```python
from build123d import *

# Parameters (mm, degrees)
SKETCH1_W           = 60
SKETCH1_H           = 20
BOSS_EXTRUDE1_DEPTH = 2.5
SKETCH2_W           = 5
SKETCH2_H           = 20
CUT_EXTRUDE1_DEPTH  = 5
CUT_EXTRUDE2_DEPTH  = 6
CUT_EXTRUDE3_DEPTH  = 6


with BuildPart() as part:
    # Sketch1 → Boss-Extrude1 (new, symmetric)
    with BuildSketch(Plane.XY):
        Rectangle(SKETCH1_W, SKETCH1_H)
    extrude(amount=BOSS_EXTRUDE1_DEPTH, both=True)

    # Sketch2 → Cut-Extrude1 (cut)
    with BuildSketch(Plane.ZY.offset(30)):
        Rectangle(SKETCH2_W, SKETCH2_H)
        with BuildLine():
            Line((1.66, 6.5), (1.66, 3.5))
            ThreePointArc((1.66, 3.5), (0, 1.84), (-1.66, 3.5))
            Line((-1.66, 3.5), (-1.66, 6.5))
            ThreePointArc((-1.66, 6.5), (0, 8.16), (1.66, 6.5))
        make_face(mode=Mode.SUBTRACT)
        with BuildLine():
            Line((1.66, -3.5), (1.66, -6.5))
            ThreePointArc((1.66, -6.5), (0, -8.16), (-1.66, -6.5))
            Line((-1.66, -6.5), (-1.66, -3.5))
            ThreePointArc((-1.66, -3.5), (0, -1.84), (1.66, -3.5))
        make_face(mode=Mode.SUBTRACT)
    extrude(amount=-CUT_EXTRUDE1_DEPTH, mode=Mode.SUBTRACT)

    # Sketch3 → Cut-Extrude2 (cut)
    with BuildSketch(Plane(origin=(30, 0, 0), x_dir=(0, 0, -1), z_dir=(1, 0, 0))):
        with BuildLine():
            Line((2.16, 3.5), (2.16, 6.5))
            ThreePointArc((2.16, 6.5), (0, 8.66), (-2.16, 6.5))
            Line((-2.16, 6.5), (-2.16, 3.5))
            ThreePointArc((-2.16, 3.5), (0, 1.34), (2.16, 3.5))
        make_face()
        with BuildLine():
            Line((2.16, -6.5), (2.16, -3.5))
            ThreePointArc((2.16, -3.5), (0, -1.34), (-2.16, -3.5))
            Line((-2.16, -3.5), (-2.16, -6.5))
            ThreePointArc((-2.16, -6.5), (0, -8.66), (2.16, -6.5))
        make_face()
    extrude(amount=-CUT_EXTRUDE2_DEPTH, mode=Mode.SUBTRACT)

    # Sketch4 → Cut-Extrude3 (cut)
    with BuildSketch(Plane(origin=(0, 0, -2.5), x_dir=(-1, 0, 0), z_dir=(0, 0, -1))):
        with BuildLine():
            Line((2.16, 6.5), (2.16, 3.5))
            ThreePointArc((2.16, 3.5), (0, 1.34), (-2.16, 3.5))
            Line((-2.16, 3.5), (-2.16, 6.5))
            ThreePointArc((-2.16, 6.5), (0, 8.66), (2.16, 6.5))
        make_face()
        with BuildLine():
            Line((-2.16, -6.5), (-2.16, -3.5))
            ThreePointArc((-2.16, -3.5), (0, -1.34), (2.16, -3.5))
            Line((2.16, -3.5), (2.16, -6.5))
            ThreePointArc((2.16, -6.5), (0, -8.66), (-2.16, -6.5))
        make_face()
    extrude(amount=-CUT_EXTRUDE3_DEPTH, mode=Mode.SUBTRACT)


solid = part.part
```
CAD build for the part. Positions are in the model's coordinates, mm. A direction names the side the tool comes from. Coordinates: 2 decimals unless noted, no trailing zeros. Loops run counter-clockwise (first coordinate to the right, second up) from the corner with the lowest first, then second, coordinate; pieces in that order, holes last. Notation, with made-up numbers: (48.5, 29) - (98.5, 29) arc R15 cw to (98.5, 38) - close; hole circle Ø8 at (20.25, 38). An arc over 180 degrees is marked (long way). Use CSV: the item, a comma, the result in double quotes. Start each with the question number.
Q1. Cut at D-D, the plane y = 7.25. List the corners of the cut face in (x, z).
Q2. Cut at C-C, the plane z = -0.7. List the corners of the cut face in (x, y).
Q3. Probe probe 1 along X at (y, z) = (3.5, 0.9); probe 2 along X at (y, z) = (-3.5, -1.85). List the from-to ranges inside material, lowest first. Write a range as from..to.
Q4. Drop flat-ended pins along their axis: P1, Ø0.9, axis at x = -28, y = 5, coming from the +Z side; P2, Ø0.9, axis at x = -28, y = 5, coming from the -Z side; P3, Ø1.3, axis at y = 5.5, z = 1, coming from the +X side. Give the stop position or say it passes through.
Q5. 3-axis set-ups, long thin cutter, end or side, ignore diameter. For faces 1 (the flat face through (-28, -5, -1.66)), 2 (the cylindrical face through (27.04, 1.34, 0.05)), 3 (the cylindrical face through (-27.54, 1.84, 0.04)), 4 (the cylindrical face through (0.05, 8.66, -0.04)): which of +Z, -Z, +X, -X, +Y, -Y reach the whole face in a straight line?
Q6. Cut at A-A, the plane x = 0. List the corners of the cut face in (y, z).
Q7. Two-plate mould, pull along Z, no slides. Class faces 5 (the flat face through (24, 5, 0)), 6 (the flat face through (-2.16, -5, 0)), 7 (the flat face through (-28, 5, -1.66)), 8 (the flat face through (-28, -5, 1.66)): +Z half, -Z half, draft (parallel to the pull), parting line (faces both ways), or undercut.
Q8. Cut at B-B, the plane y = -4.25. List the corners of the cut face in (x, z).
Here are the results:
1,outline,"(-30, -1.48) - (-25, -1.48) - (-25, -2.5) - (-2.03, -2.5) - (-2.03, 2.5) - (-25, 2.5) - (-25, 1.48) - (-30, 1.48) - close; (2.03, -2.5) - (30, -2.5) - (30, -2.03) - (24, -2.03) - (24, 2.03) - (30, 2.03) - (30, 2.5) - (2.03, 2.5) - close"
2,outline,"(-30, -8.01) - (-25, -8.01) - (-25, -10) - (30, -10) - (30, -8.54) - (24, -8.54) - (24, -1.46) - (30, -1.46) - (30, 1.46) - (24, 1.46) - (24, 8.54) - (30, 8.54) - (30, 10) - (-25, 10) - (-25, 8.01) - (-30, 8.01) - (-30, 1.99) - (-25, 1.99) - (-25, -1.99) - (-30, -1.99) - close; hole (-2.16, -6.5) arc R2.16 ccw to (2.16, -6.5) - (2.16, -3.5) arc R2.16 ccw to (-2.16, -3.5) - close; hole (-2.16, 3.5) arc R2.16 ccw to (2.16, 3.5) - (2.16, 6.5) arc R2.16 ccw to (-2.16, 6.5) - close"
3,probe 1,"-30..-2.16, 2.16..24"
3,probe 2,"-25..-2.16, 2.16..24"
4,P1,"z = 1.66"
4,P2,"z = -1.66"
4,P3,"x = 24"
5,face 1,"-Z, -X, +Y, -Y"
5,face 2,"+X"
5,face 3,"-X"
5,face 4,"+Z, -Z"
6,outline,"(-10, -2.5) - (-8.66, -2.5) - (-8.66, 2.5) - (-10, 2.5) - close; (-1.34, -2.5) - (1.34, -2.5) - (1.34, 2.5) - (-1.34, 2.5) - close; (8.66, -2.5) - (10, -2.5) - (10, 2.5) - (8.66, 2.5) - close"
7,face 5,"undercut"
7,face 6,"draft"
7,face 7,"-Z half"
7,face 8,"+Z half"
8,outline,"(-30, -1.66) - (-25, -1.66) - (-25, -2.5) - (-2.16, -2.5) - (-2.16, 2.5) - (-25, 2.5) - (-25, 1.66) - (-30, 1.66) - close; (2.16, -2.5) - (30, -2.5) - (30, -2.16) - (24, -2.16) - (24, 2.16) - (30, 2.16) - (30, 2.5) - (2.16, 2.5) - close"
